from build123d import *

# Parameters (mm, degrees)
SKETCH1_R           = 1.5
SKETCH1_W           = 4
SKETCH1_H           = 10
BOSS_EXTRUDE1_DEPTH = 4


with BuildPart() as part:
    # Sketch1 → Boss-Extrude1 (new body)
    with BuildSketch(Plane(origin=(0, 0, 0), x_dir=(1, 0, 0), z_dir=(0, 1, 0))):
        with BuildLine():
            ThreePointArc((-5.484552972, 0.411920736), (0, -5.5), (5.484552972, 0.411920736))
            ThreePointArc((5.484552972, 0.411920736), (4.75, 20), (5.484552972, 39.588079264))
            ThreePointArc((5.484552972, 39.588079264), (5.499845666, 39.95879751), (5.490108902, 40.329703267))
            ThreePointArc((5.490108902, 40.329703267), (4.75, 65), (5.490108902, 89.670296733))
            ThreePointArc((5.490108902, 89.670296733), (0, 95.5), (-5.490108902, 89.670296733))
            ThreePointArc((-5.490108902, 89.670296733), (-4.75, 65), (-5.490108902, 40.329703267))
            ThreePointArc((-5.490108902, 40.329703267), (-5.499845666, 39.95879751), (-5.484552972, 39.588079264))
            ThreePointArc((-5.484552972, 39.588079264), (-4.75, 20), (-5.484552972, 0.411920736))
        make_face()
        Circle(SKETCH1_R, mode=Mode.SUBTRACT)
        with Locations((0, 90)):
            Circle(SKETCH1_R, mode=Mode.SUBTRACT)
        with Locations((0, 40)):
            Circle(SKETCH1_R, mode=Mode.SUBTRACT)
        with Locations((0, 61.5)):
            Rectangle(SKETCH1_W, SKETCH1_H, mode=Mode.SUBTRACT)
    extrude(amount=BOSS_EXTRUDE1_DEPTH)


solid = part.part
Geometry check sheet. Reference: the model listing, model coordinates, mm. A direction names the side the tool comes from. Round coordinates to 2 decimals unless told otherwise and drop trailing zeros. Write each loop counter-clockwise with the first axis right and the second up, starting at its lowest first coordinate (ties: lowest second). Pieces come first, ordered by that corner, then holes. Notation, with made-up numbers: (-1.5, 20) - (56.5, 20) arc R34 cw to (56.5, 50) - close; hole circle Ø6 at (10, 13.5). An arc over 180 degrees is marked (long way). One line per item, written item: value.
1. Scan lines: L1, parallel to Z at x = 0.5, y = 1.6; L2, parallel to X at y = 3.25, z = -90; L3, parallel to X at y = 2, z = -91. Record each from-to range of solid material in increasing order.
The answers:
L1: z = -95.48 to -91.41, -88.59 to -66.5, -56.5 to -41.41, -38.59 to -1.41, 1.41 to 5.48
L2: x = -5.5 to -1.5, 1.5 to 5.5
L3: x = -5.41 to -1.12, 1.12 to 5.41
2. Set-up check for faces 5 (the face through (4.75, 1.97, -19.73)), 6 (the face through (-2, 2, -61)): record each of +Z, -Z, +X, -X, +Y, -Y from which the full face is reachable in a straight line by a thin tool's end or side.
The answers:
face 5: +X, +Y, -Y
face 6: +Y, -Y
3. Cross-section at C-C on x = -3.75. Record the boundary of the cut face in (y, z), and give its area (3 significant figures).
The answers:
outline: (0, -94.02) - (4, -94.02) - (4, 4.02) - (0, 4.02) - close
area: 392 mm^2
4. Depth check by flat-ended pin: pin 1 Ø3.5 at (x, z) = (0, 0) entering from +Y; pin 2 Ø2 at (x, y) = (2.5, 2.5) entering from -Z; pin 3 Ø2 at (y, z) = (3.5, -29.5) entering from -X; pin 4 Ø2 at (y, z) = (1, -59.5) entering from +X. Enter the tip coordinate at first touch or a pass-through.
The answers:
pin 1: stops at y = 4
pin 2: stops at z = -95.29
pin 3: stops at x = -4.96
pin 4: stops at x = 4.8
5. Cross-section at D-D on z = -13.5. Record the boundary of the cut face in (x, y), and give its area (3 significant figures).
The answers:
outline: (-4.83, 0) - (4.83, 0) - (4.83, 4) - (-4.83, 4) - close
area: 38.6 mm^2
6. Mould release check, pull along X, two halves, no side actions. Record for faces 1 (the face through (-4.75, 1.97, -20.27)), 2 (the face through (-0.325, 1.972, -38.536)), 3 (the face through (0, 0, -46)), 4 (the face through (4.75, 1.97, -64.65)): released by +X, released by -X, zero draft, split by the parting line, or undercut.
The answers:
face 1: released by -X
face 2: undercut
face 3: zero draft
face 4: released by +X
7. Cross-section at B-B on z = -64.5. Record the boundary of the cut face in (x, y), and give its area (3 significant figures).
The answers:
outline: (-4.75, 0) - (-2, 0) - (-2, 4) - (-4.75, 4) - close; (2, 0) - (4.75, 0) - (4.75, 4) - (2, 4) - close
area: 22.0 mm^2
8. Cross-section at A-A on y = 0.7. Record the boundary of the cut face in (x, z).
The answers:
outline: (-5.49, -89.67) arc R5.5 ccw (long way) to (5.49, -89.67) arc R411.54 cw to (5.49, -40.33) arc R5.5 ccw to (5.48, -39.59) arc R261.54 cw to (5.48, -0.41) arc R5.5 ccw (long way) to (-5.48, -0.41) arc R261.54 cw to (-5.48, -39.59) arc R5.5 ccw to (-5.49, -40.33) arc R411.54 cw to start; hole (-2, -66.5) - (2, -66.5) - (2, -56.5) - (-2, -56.5) - close; hole circle Ø3 at (0, -90); hole circle Ø3 at (0, -40); hole circle Ø3 at (0, 0)
